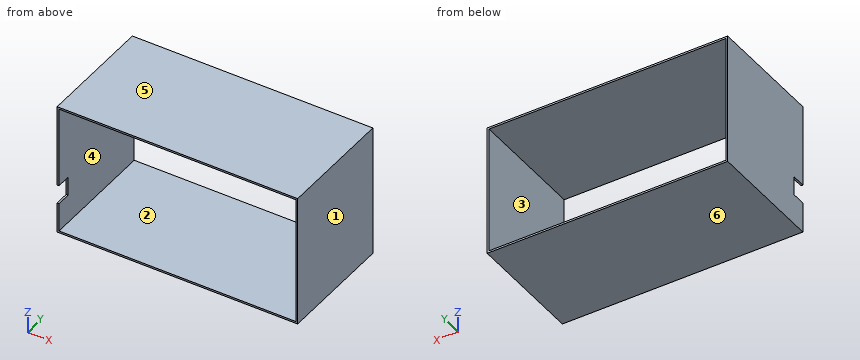
```python
from build123d import *

# Parameters (mm, degrees)
SKETCH1_W      = 102
SKETCH1_H      = 56
SKETCH1_W_2    = 100.4
SKETCH1_H_2    = 54.4
WALLS_DEPTH    = 50
USB_HOLE_REACH = 118.996
SKETCH3_W      = 8
SKETCH3_H      = 6


with BuildPart() as part:
    # Sketch1 → WALLS (new body)
    with BuildSketch(Plane(origin=(0, 0, 0), x_dir=(1, 0, 0), z_dir=(0, 1, 0))):
        Rectangle(SKETCH1_W, SKETCH1_H)
        Rectangle(SKETCH1_W_2, SKETCH1_H_2, mode=Mode.SUBTRACT)
    extrude(amount=WALLS_DEPTH)

    # Sketch3 → USB_HOLE (cut, up to next)
    with BuildSketch(Plane.ZY.offset(51), mode=Mode.PRIVATE) as usb_hole_sk1:
        with Locations((-11, 3)):
            Rectangle(SKETCH3_W, SKETCH3_H)
    usb_hole_tool1 = extrude(usb_hole_sk1.sketch, amount=-USB_HOLE_REACH, mode=Mode.PRIVATE) & part.part
    add(usb_hole_tool1.solids().sort_by_distance((-51, 3, -11))[0], mode=Mode.SUBTRACT)


solid = part.part
```
Check sheet for the modelled part. Datum: model origin and axes. Units: mm. Face numbers are marked on the shaded views. A direction names the side the tool comes from. Round coordinates to 2 decimals unless told otherwise and drop trailing zeros. Loops run counter-clockwise (first coordinate to the right, second up) from the corner with the lowest first, then second, coordinate; pieces in that order, holes last. Notation, with made-up numbers: (80, 29.5) - (101, 29.5) arc R24 cw to (101, 67.5) - close; hole circle Ø4 at (30.5, -36). An arc over 180 degrees is marked (long way). Answer as a JSON object with one key per item and string values. Group by question number.
Q1. Mould release check, pull along Z, two halves, no side actions. Record for the marked faces 3, 4, 5 and 6: released by +Z, released by -Z, zero draft, split by the parting line, or undercut.
Q2. Sectioned sample at A-A, the plane z = 18. Enter the section's corners in (x, y), plus the area to 3 significant figures.
Q3. Set-up check for the marked faces 1 and 2: record each of +Z, -Z, +X, -X, +Y, -Y from which the full face is reachable in a straight line by a thin tool's end or side.
Q4. Sectioned sample at B-B, the plane x = -4.5. Enter the section's corners in (y, z).
Q5. Sectioned sample at C-C, the plane y = 39. Enter the section's corners in (x, z).
Q6. Scan lines: line 1 along Z through (x, y) = (-4.5, 37); line 2 along X through (y, z) = (48, -17.5). Record each from-to range of solid material in increasing order. Write a range as [from, to].
Q7. Gauge pin test, flat end, axial feed: P1, Ø0.6, axis at x = -50.5, z = -11.5, coming from the -Y side. Record the tip position at first contact, or that the pin passes through.
Solution:
{
 "1": {"face 3": "undercut", "face 4": "undercut", "face 5": "released by +Z", "face 6": "released by -Z"},
 "2": {"outline": "(-51, 0) - (-50.2, 0) - (-50.2, 50) - (-51, 50) - close; (50.2, 0) - (51, 0) - (51, 50) - (50.2, 50) - close", "area": "80.0 mm²"},
 "3": {"face 1": "+Z, -Z, +X, +Y, -Y", "face 2": "+Y, -Y"},
 "4": {"outline": "(0, -28) - (50, -28) - (50, -27.2) - (0, -27.2) - close; (0, 27.2) - (50, 27.2) - (50, 28) - (0, 28) - close"},
 "5": {"outline": "(-51, -28) - (51, -28) - (51, 28) - (-51, 28) - close; hole (-50.2, -27.2) - (50.2, -27.2) - (50.2, 27.2) - (-50.2, 27.2) - close"},
 "6": {"line 1": "z = [-28, -27.2], [27.2, 28]", "line 2": "x = [-51, -50.2], [50.2, 51]"},
 "7": {"P1": "stops at y = 6"}
}
